from build123d import *

# Parameters (mm, degrees)
IZIM2_R                     = 13
IZIM2_W                     = 70
IZIM2_H                     = 72
Y_KSEKLIK_EKSTR_ZYON1_DEPTH = 34
IZIM3_OUTSIDE_W             = 181.26
IZIM3_OUTSIDE_H             = 69.26
KES_EKSTR_ZYON4_DEPTH       = 73


with BuildPart() as part:
    # Çizim2 → Yükseklik-Ekstrüzyon1 (new body)
    with BuildSketch(Plane(origin=(0, 0, 0), x_dir=(1, 0, 0), z_dir=(0, 1, 0))):
        with BuildLine():
            Line((35, 36), (35, -36))
            Line((35, -36), (75, -36))
            ThreePointArc((75, -36), (111, 0), (75, 36))
            Line((75, 36), (35, 36))
        make_face()
        with Locations((75, 0)):
            Circle(IZIM2_R, mode=Mode.SUBTRACT)
        Rectangle(IZIM2_W, IZIM2_H)
        Circle(IZIM2_R, mode=Mode.SUBTRACT)
    extrude(amount=-Y_KSEKLIK_EKSTR_ZYON1_DEPTH)

    # Çizim3 outside → Kes-Ekstrüzyon4 (cut, through all)
    with BuildSketch(Plane.XY.offset(36)):
        with Locations((38, -17)):
            Rectangle(IZIM3_OUTSIDE_W, IZIM3_OUTSIDE_H)
        Polygon((-35, 0), (-35, -34), (-20, -34), (-20, -16), (20, -16), (20, -34), (75, -34), (111, -34), (111, -20), (75, -20), (35, -20), (35, 0), align=None, mode=Mode.SUBTRACT)
    extrude(amount=-KES_EKSTR_ZYON4_DEPTH, mode=Mode.SUBTRACT)


solid = part.part
Geometry: final body of the model. Coordinates: model frame, mm. A direction names the side the tool comes from. Coordinates: 2 decimals unless noted, no trailing zeros. Order: outer loops, then holes, each group sorted by start corner. A loop starts at its lowest first (then second) coordinate and runs counter-clockwise, first axis right, second up. Notation, with made-up numbers: M -20,83.5 L 29,83.5 A19 ccw 29,89.5 Z; hole C 61,60.5 d1. An arc over 180 degrees is marked long. One line per question, with ' | ' between items. Start each with the question number.
Item 1: Pin query (flat end, axial travel): pin 1 Ø21.5 at (x, z) = (90, -14.5) entering from +Y; pin 2 Ø8 at (x, z) = (-7, 15) entering from -Y; pin 3 Ø9 at (y, z) = (-25.5, -12.5) entering from +X; pin 4 Ø23.5 at (x, z) = (75, 0) entering from +Y. Return the tip coordinate at first contact, or that it passes through.
Item 2: Cut plane D-D, the plane y = -11.5. Return the cut outline in (x, z).
Item 3: Draft query along Z for faces 1 (the flat face through (20, -25, 1)), 2 (the cylindrical face through (62.013, -26.902, -0.572)), 3 (the flat face through (19, -13, 36)). Return one class per face: released by +Z, released by -Z, zero draft, split by the parting line, or undercut.
Item 4: Cut plane A-A, the plane y = -24.5. Return the cut outline in (x, z).
Item 5: Cut plane C-C, the plane x = 0. Return the cut outline in (y, z), then the cut area to 3 significant figures.
Item 6: Cut plane B-B, the plane z = 0. Return the cut outline in (x, y), then the cut area to 3 significant figures.
Item 7: Ray query, probe 1 along X at (y, z) = (-25, 0); probe 2 along X at (y, z) = (-7.25, 0); probe 3 along Z at (x, y) = (75, -27.75). Return the intervals inside material, ascending. Write a range as [from, to].
Item 8: Set-up query: faces 4 (the cylindrical face through (110.99, -26.9, 0.79)), 5 (the flat face through (-14, -16, 1)), 6 (the flat face through (64, -20, 9)). Return all of +Z, -Z, +X, -X, +Y, -Y with unobstructed straight access to the full face (end or side cutting, diameter ignored); none if empty.
A:
1) pin 1: stops at y = -20 | pin 2: stops at y = -16 | pin 3: stops at x = 110.1 | pin 4: passes through
2) outline: M -35,-36 L 35,-36 L 35,36 L -35,36 Z; hole C 0,0 d26
3) face 1: zero draft | face 2: undercut | face 3: released by +Z
4) outline: M -35,-36 L -20,-36 L -20,36 L -35,36 Z; M 20,-36 L 75,-36 A36 ccw 75,36 L 20,36 Z; hole C 75,0 d26
5) outline: M -16,-36 L 0,-36 L 0,-13 L -16,-13 Z; M -16,13 L 0,13 L 0,36 L -16,36 Z | area: 736 mm2
6) outline: M -35,-34 L -20,-34 L -20,-16 L -13,-16 L -13,0 L -35,0 Z; M 13,-16 L 20,-16 L 20,-34 L 62,-34 L 62,-20 L 35,-20 L 35,0 L 13,0 Z; M 88,-34 L 111,-34 L 111,-20 L 88,-20 Z | area: 1,940 mm2
7) probe 1: x = [-35, -20], [20, 62], [88, 111] | probe 2: x = [-35, -13], [13, 35] | probe 3: z = [-36, -13], [13, 36]
8) face 4: +X, +Y, -Y | face 5: +Z, -Z, -Y | face 6: +Z, -Z, +X, +Y
